Read the model definition and answer for the solid it produces. Units are mm, in the model's axes. Face numbers are marked on the shaded views. A direction names the side the tool comes from. Round coordinates to 2 decimals unless told otherwise and drop trailing zeros. Order: outer loops, then holes, each group sorted by start corner. A loop starts at its lowest first (then second) coordinate and runs counter-clockwise, first axis right, second up. Notation, with made-up numbers: (50.25, -19.5) - (73.25, -19.5) arc R17 cw to (73.25, -9.5) - close; hole circle Ø1 at (47.5, 63). An arc over 180 degrees is marked (long way). Put each result on its own line as item: value. Start each with the question number.
Q1. Each of these flat-tipped pins is pushed along its axis until it touches: pin 1 Ø2 at (x, y) = (21, 8.5) entering from -Z; pin 2 Ø2.5 at (y, z) = (9.5, -5) entering from +X; pin 3 Ø5.5 at (y, z) = (7, -22) entering from -X. Where does it stop, or does it pass through?
Q2. Section C-C on y = 7.5 is taken. Give the vertices of the cut face in (x, z), then the cut area to 3 significant figures.
Q3. Which of the six approach directions +Z, -Z, +X, -X, +Y, -Y give full straight-line access (tool end or side, diameter ignored) to the marked faces 1, 2 and 3?
Q4. Section D-D on x = 25 is taken. Give the vertices of the cut face in (y, z), then the cut area to 3 significant figures.
Q5. Find the intervals of material crossed by line 1 along X through (y, z) = (0.65, -4); line 2 along Z through (x, y) = (13, 18); line 3 along Y through (x, z) = (9, -19.5), in increasing order. Write a range as from..to.
Q6. Section B-B on z = -4.5 is taken. Give the vertices of the cut face in (x, y), then the cut area to 3 significant figures.
Q7. Section A-A on x = 4 is taken. Give the vertices of the cut face in (y, z), then the cut area to 3 significant figures.
from build123d import *

# Parameters (mm, degrees)
SKETCH2_W           = 50
SKETCH2_H           = 27.5
SKETCH2_R           = 1.6
BOSS_EXTRUDE1_DEPTH = 1.5
FILLET1_R           = 3
SKETCH3_W           = 10
SKETCH3_H           = 10
BOSS_EXTRUDE2_DEPTH = 19


with BuildPart() as part:
    # Sketch2 → Boss-Extrude1 (new body)
    with BuildSketch(Plane(origin=(0, 0, 0), x_dir=(1, 0, 0), z_dir=(0, 1, 0))):
        with Locations((25, 13.75)):
            Rectangle(SKETCH2_W, SKETCH2_H)
        with Locations(Location((46, 23.5, 0), (0, 0, 270))):
            Circle(SKETCH2_R, mode=Mode.SUBTRACT)
        with Locations(Location((46, 4, 0), (0, 0, 270))):
            Circle(SKETCH2_R, mode=Mode.SUBTRACT)
        with Locations(Location((4, 23.5, 0), (0, 0, 270))):
            Circle(SKETCH2_R, mode=Mode.SUBTRACT)
        with Locations(Location((4, 4, 0), (0, 0, 270))):
            Circle(SKETCH2_R, mode=Mode.SUBTRACT)
    extrude(amount=BOSS_EXTRUDE1_DEPTH)

    # Fillet1
    fillet1_edges = [part.edges().sort_by_distance(p)[0] for p in [
        (0, 0.75, 0),
        (0, 0.75, -27.5),
        (50, 0.75, -27.5),
        (50, 0.75, 0),
    ]]
    fillet(fillet1_edges, radius=FILLET1_R)

    # Sketch3 → Boss-Extrude2 (add)
    with BuildSketch(Plane(origin=(0, 0, 0), x_dir=(1, 0, 0), z_dir=(0, 1, 0))):
        with Locations((5, 13.75)):
            Rectangle(SKETCH3_W, SKETCH3_H)
        Polygon((10, 18.75), (10, 8.75), (10, 3.75), (40, 3.75), (40, 8.75), (40, 18.75), (40, 23.75), (10, 23.75), align=None)
        with Locations((45, 13.75)):
            Rectangle(SKETCH3_W, SKETCH3_H)
    extrude(amount=BOSS_EXTRUDE2_DEPTH)


solid = part.part
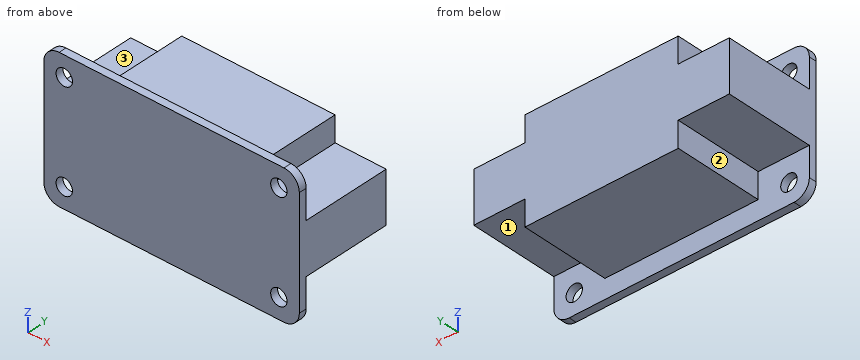
Findings:
1. pin 1: z = -23.75
1. pin 2: x = 40
1. pin 3: x = 10
2. outline: (0, -18.75) - (10, -18.75) - (10, -23.75) - (40, -23.75) - (40, -18.75) - (50, -18.75) - (50, -8.75) - (40, -8.75) - (40, -3.75) - (10, -3.75) - (10, -8.75) - (0, -8.75) - close
2. area: 800 mm2
3. face 1: -Z, +X, +Y
3. face 2: -Z, -X, +Y
3. face 3: +Z, -X, +Y
4. outline: (0, -27.5) - (1.5, -27.5) - (1.5, -23.75) - (19, -23.75) - (19, -3.75) - (1.5, -3.75) - (1.5, 0) - (0, 0) - close
4. area: 391 mm2
5. line 1: 0..2.4, 5.6..44.4, 47.6..50
5. line 2: -23.75..-3.75
5. line 3: 0..1.5
6. outline: (0, 0) - (2.48, 0) - (2.48, 1.5) - (0, 1.5) - close; (5.52, 0) - (44.48, 0) - (44.48, 1.5) - (40, 1.5) - (40, 19) - (10, 19) - (10, 1.5) - (5.52, 1.5) - close; (47.52, 0) - (50, 0) - (50, 1.5) - (47.52, 1.5) - close
6. area: 591 mm2
7. outline: (0, -27.5) - (1.5, -27.5) - (1.5, -25.1) - (0, -25.1) - close; (0, -21.9) - (1.5, -21.9) - (1.5, -18.75) - (19, -18.75) - (19, -8.75) - (1.5, -8.75) - (1.5, -5.6) - (0, -5.6) - close; (0, -2.4) - (1.5, -2.4) - (1.5, 0) - (0, 0) - close
7. area: 207 mm2
